```python
from build123d import *

# Parameters (mm, degrees)
SKETCH1_W           = 73
SKETCH1_H           = 60
SKETCH1_R           = 26.1
BOSS_EXTRUDE1_DEPTH = 16
BOSS_EXTRUDE2_START = -7
SKETCH3_R           = 26.1
SKETCH3_R_2         = 24
BOSS_EXTRUDE2_DEPTH = 2
SKETCH2_R           = 1.5
CUT_EXTRUDE1_DEPTH  = 15
CUT_EXTRUDE2_START  = -73
SKETCH2_2_R         = 1.5
CUT_EXTRUDE2_DEPTH  = 15


with BuildPart() as part:
    # Sketch1 → Boss-Extrude1 (new body)
    with BuildSketch(Plane(origin=(0, 0, 0), x_dir=(1, 0, 0), z_dir=(0, 1, 0))):
        with Locations((36.5, 30)):
            Rectangle(SKETCH1_W, SKETCH1_H)
        with Locations((36.5, 30)):
            Circle(SKETCH1_R, mode=Mode.SUBTRACT)
    extrude(amount=BOSS_EXTRUDE1_DEPTH)

    # Sketch3 → Boss-Extrude2 (add)
    with BuildSketch(Plane(origin=(0, 16, 0), x_dir=(1, 0, 0), z_dir=(0, 1, 0)).offset(BOSS_EXTRUDE2_START)):
        with Locations((36.5, 30)):
            Circle(SKETCH3_R)
        with Locations((36.5, 30)):
            Circle(SKETCH3_R_2, mode=Mode.SUBTRACT)
    extrude(amount=-BOSS_EXTRUDE2_DEPTH)

    # Sketch2 → Cut-Extrude1 (cut)
    with BuildSketch(Plane(origin=(73, 0, 0), x_dir=(0, 0, -1), z_dir=(1, 0, 0))):
        with Locations((10, 8)):
            Circle(SKETCH2_R)
        with Locations((50, 8)):
            Circle(SKETCH2_R)
    extrude(amount=-CUT_EXTRUDE1_DEPTH, mode=Mode.SUBTRACT)

    # Sketch2<2> → Cut-Extrude2 (cut)
    with BuildSketch(Plane(origin=(73, 0, 0), x_dir=(0, 0, -1), z_dir=(1, 0, 0)).offset(CUT_EXTRUDE2_START)):
        with Locations((10, 8)):
            Circle(SKETCH2_2_R)
        with Locations((50, 8)):
            Circle(SKETCH2_2_R)
    extrude(amount=CUT_EXTRUDE2_DEPTH, mode=Mode.SUBTRACT)


solid = part.part
```
Input: part model. Units: mm. Frame: model coordinates. A direction names the side the tool comes from. Round coordinates to 2 decimals unless told otherwise and drop trailing zeros. Loops run counter-clockwise (first coordinate to the right, second up) from the corner with the lowest first, then second, coordinate; pieces in that order, holes last. Notation, with made-up numbers: (43, 78) - (81, 78) arc R9 ccw to (81, 86) - close; hole circle Ø9 at (38.25, 81). An arc over 180 degrees is marked (long way). One line per item, written item: value. Start each with the question number.
(1) Ray query, line 1 (X direction, y = 13.75, z = -30); line 2 (Y direction, x = 4, z = -10); line 3 (X direction, y = 8, z = -30). Return the intervals inside material, ascending. Write a range as [from, to].
(2) Draft query along Z for faces 1 (the flat face through (19.8, 0, -50.4)), 2 (the flat face through (58, 8, -10)), 3 (the cylindrical face through (7.4, 7.1, -8.8)), 4 (the flat face through (36, 8, 0)). Return one class per face: +Z half, -Z half, draft (parallel to the pull), parting line (faces both ways), or undercut.
(3) Section B-B, the plane z = -30. Return loops of the section in (x, y).
(4) Section D-D, the plane y = 2. Return loops of the section in (x, z), plus the area to 3 significant figures.
(5) Section A-A, the plane x = 59. Return loops of the section in (y, z).
(6) Contact query for flat-ended pins moving along their axis: P1, Ø1.5, axis at y = 8, z = -10.5, coming from the -X side; P2, Ø0.9, axis at y = 8.5, z = -10, coming from the +X side; P3, Ø6, axis at x = 42.5, y = 3, coming from the +Z side; P4, Ø4, axis at x = 43.5, z = -9, coming from the -Y side. Output: stop coordinate, or through.
(7) Access query for faces 5 (the cylindrical face through (30.84, 12.45, -4.52)), 6 (the flat face through (58, 7, -19)), 7 (the flat face through (15, 8, -10)), 8 (the cylindrical face through (65.6, 7.1, -8.8)), 9 (the flat face through (36, 8, -60)). Directions: +Z, -Z, +X, -X, +Y, -Y. A direction counts if a zero-diameter tool reaches every point of the face in a straight line with its end or side. Return the directions, or none.
(8) Section C-C, the plane x = 37.5. Return loops of the section in (y, z), plus the area to 3 significant figures.
Results below:
1. line 1: [0, 10.4], [62.6, 73]
1. line 2: [0, 6.5], [9.5, 16]
1. line 3: [0, 12.5], [60.5, 73]
2. face 1: draft
2. face 2: undercut
2. face 3: undercut
2. face 4: +Z half
3. outline: (0, 0) - (10.4, 0) - (10.4, 7) - (12.5, 7) - (12.5, 9) - (10.4, 9) - (10.4, 16) - (0, 16) - close; (60.5, 7) - (62.6, 7) - (62.6, 0) - (73, 0) - (73, 16) - (62.6, 16) - (62.6, 9) - (60.5, 9) - close
4. outline: (0, -60) - (73, -60) - (73, 0) - (0, 0) - close; hole circle Ø52.2 at (36.5, -30)
4. area: 2,240 mm^2
5. outline: (0, -60) - (16, -60) - (16, -43.23) - (9, -43.23) - (9, -38.35) - (7, -38.35) - (7, -43.23) - (0, -43.23) - close; (0, -16.77) - (7, -16.77) - (7, -21.65) - (9, -21.65) - (9, -16.77) - (16, -16.77) - (16, 0) - (0, 0) - close; hole circle Ø3 at (8, -50); hole circle Ø3 at (8, -10)
6. P1: x = 15
6. P2: x = 58
6. P3: z = 0
6. P4: y = 7
7. face 5: +Y
7. face 6: -Y
7. face 7: -X
7. face 8: +X
7. face 9: -Z, +X, -X, +Y, -Y
8. outline: (0, -60) - (16, -60) - (16, -56.08) - (9, -56.08) - (9, -53.98) - (7, -53.98) - (7, -56.08) - (0, -56.08) - close; (0, -3.92) - (7, -3.92) - (7, -6.02) - (9, -6.02) - (9, -3.92) - (16, -3.92) - (16, 0) - (0, 0) - close
8. area: 134 mm^2
